Work out the finished part from the listing and answer in its coordinate system (mm). Give positions to 0.01 mm unless a question says otherwise; leave off trailing zeros. Loops run counter-clockwise (first coordinate to the right, second up) from the corner with the lowest first, then second, coordinate; pieces in that order, holes last. Notation, with made-up numbers: (-30.5, 84.25) -> (-16.5, 84.25) arc R33 ccw to (-16.5, 121.25) -> close; hole circle Ø6 at (4, -15.5). An arc over 180 degrees is marked (long way). Answer as CSV lines item,"result". Start each with the question number.
1. Flat-ended cylindrical pins translate along their axes: pin 1 Ø1.5 at (y, z) = (2, -79.5) entering from +X; pin 2 Ø3 at (y, z) = (11.5, -137) entering from -X; pin 3 Ø3 at (x, z) = (-8, -103.5) entering from -Y. Find the tip coordinate at first contact, or state that the pin passes through.
2. Find section B-B, the plane z = -152. Give the vertices of the cut face in (x, y) (1 decimal).
3. Find the intervals of material crossed by line 1 along Y through (x, z) = (-19.5, -167); line 2 along Y through (x, z) = (-7.75, -172); line 3 along X through (y, z) = (2.25, -194), in increasing order.
4. Find section A-A, the plane x = -10. Give the vertices of the cut face in (y, z) (3 decimals), and give its area (3 significant figures).
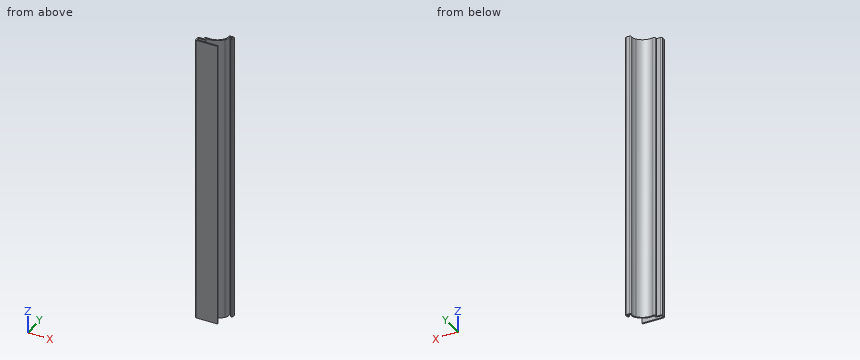
from build123d import *

# Parameters (mm, degrees)
EXTRUDE_THIN1_DEPTH = 206.375
FILLET1_R           = 1.016


with BuildPart() as part:
    # Sketch1 → Extrude-Thin1 (new body)
    with BuildSketch(Plane.XY):
        with BuildLine():
            Line((-0.79375, 11.731625), (0, 14.906625))
            Line((0, 14.906625), (-4.7625, 14.906625))
            ThreePointArc((-4.7625, 14.906625), (-4.309569444, 12.373308652), (-5.240769358, 9.974203708))
            ThreePointArc((-5.240769358, 9.974203708), (-10.374425557, 6.332169642), (-16.66875, 6.35))
            Line((-16.66875, 6.35), (-16.66875, 3.96875))
            Line((-16.66875, 3.96875), (-20.6375, 3.96875))
            Line((-20.6375, 3.96875), (-20.6375, 0))
            Line((-20.6375, 0), (-4.7625, 0.396875))
            Line((-4.7625, 0.396875), (-4.787892066, 1.412557649))
            Line((-4.787892066, 1.412557649), (-19.6215, 1.04171745))
            Line((-19.6215, 1.04171745), (-19.6215, 2.95275))
            Line((-19.6215, 2.95275), (-15.65275, 2.95275))
            Line((-15.65275, 2.95275), (-15.65275, 5.040913964))
            ThreePointArc((-15.65275, 5.040913964), (-9.419658883, 5.590889524), (-4.428168187, 9.364338693))
            ThreePointArc((-4.428168187, 9.364338693), (-3.423343097, 11.516274139), (-3.36895913, 13.890625))
            Line((-3.36895913, 13.890625), (-1.301268829, 13.890625))
            Line((-1.301268829, 13.890625), (-1.77941478, 11.978041195))
            Line((-1.77941478, 11.978041195), (-0.79375, 11.731625))
        make_face()
    extrude(amount=-EXTRUDE_THIN1_DEPTH)

    # Fillet1
    fillet1_edges = [part.edges().sort_by_distance(p)[0] for p in [
        (-20.6375, 0, -103.1875),
        (-20.6375, 3.96875, -103.1875),
        (-16.66875, 6.35, -103.1875),
        (-4.7625, 14.906625, -103.1875),
        (0, 14.906625, -103.1875),
        (-15.65275, 2.95275, -103.1875),
    ]]
    fillet(fillet1_edges, radius=FILLET1_R)


solid = part.part
Resolved:
1,pin 1,"stops at x = -4.78"
1,pin 2,"stops at x = -5.22"
1,pin 3,"stops at y = 0.28"
2,outline,"(-20.6, 1) arc R1 ccw to (-19.6, 0) -> (-4.8, 0.4) -> (-4.8, 1.4) -> (-19.6, 1) -> (-19.6, 3) -> (-16.7, 3) arc R1 ccw to (-15.7, 4) -> (-15.7, 5) arc R11.3 ccw to (-4.4, 9.4) arc R5.8 ccw to (-3.4, 13.9) -> (-1.3, 13.9) -> (-1.8, 12) -> (-0.8, 11.7) -> (-0.3, 13.6) arc R1 ccw to (-1.3, 14.9) -> (-3.4, 14.9) arc R1 ccw to (-4.4, 13.7) arc R4.8 cw to (-5.2, 10) arc R10.3 cw to (-15.5, 6) arc R1 ccw to (-16.7, 5) -> (-16.7, 4) -> (-19.6, 4) arc R1 ccw to (-20.6, 3) -> close"
3,line 1,"y = 0.03 to 1.04, 2.95 to 3.97"
3,line 2,"y = 0.32 to 1.34, 6.4 to 7.6"
3,line 3,"x = -20.64 to -19.62"
4,outline,"(0.266, -206.375) -> (1.282, -206.375) -> (1.282, 0) -> (0.266, 0) -> close; (5.385, -206.375) -> (6.459, -206.375) -> (6.459, 0) -> (5.385, 0) -> close"
4,area,"431 mm^2"
